Part model, mm, in its own coordinate system. A direction names the side the tool comes from. Round coordinates to 2 decimals unless told otherwise and drop trailing zeros. Loops run counter-clockwise (first coordinate to the right, second up) from the corner with the lowest first, then second, coordinate; pieces in that order, holes last. Notation, with made-up numbers: (78.25, 17) - (123.25, 17) arc R32 ccw to (123.25, 50) - close; hole circle Ø9 at (47, -8). An arc over 180 degrees is marked (long way). Write each question's results on one line, items separated by ' | '. Start each with the question number.
(1) Mould opens along X. For faces 4 (the face through (-90.49, -63, 1)), 5 (the face through (-105, -85.722, 1)), 6 (the face through (-107.615, -92, 1)) say: released by +X, released by -X, zero draft, split by the parting line, or undercut.
(2) Cut at A-A, the plane x = -114. List the corners of the cut face in (y, z), then the cut area to 3 significant figures.
(3) Cut at B-B, the plane y = -76. List the corners of the cut face in (x, z).
(4) Cut at D-D, the plane x = -88. List the corners of the cut face in (y, z).
(5) Cut at C-C, the plane z = 2. List the corners of the cut face in (x, y).
(6) Flat gauge pins, fed straight in: P1, Ø1.2, axis at x = -100.5, z = 1.5, coming from the +Y side; P2, Ø3, axis at x = -116.5, y = -84.5, coming from the -Z side; P3, Ø1.2, axis at y = -92.5, z = 1, coming from the +X side; P4, Ø1.2, axis at y = -91.5, z = 1.5, coming from the -X side. Where does each tip first touch, or does it go through?
(7) Tool access for faces 1 (the face through (-107.615, -63, 1)), 2 (the face through (-120.38, -70.12, 1.22)), 3 (the face through (-116, -90.722, 1)): list every direction of +Z, -Z, +X, -X, +Y, -Y with a clear straight run to the whole face (end or side of a thin tool).
(8) Drill centre lines: L1, parallel to Y at x = -98, z = 1.6; L2, parallel to X at y = -78, z = 1.8; L3, parallel to Y at x = -107.5, z = 2.25. Where is each one in solid material? Low to high.
from build123d import *

# Parameters (mm, degrees)
SALIENTE_EXTRUIR1_DEPTH = 2.4
CORTAR_EXTRUIR1_DEPTH   = 4


with BuildPart() as part:
    # Croquis1 → Saliente-Extruir1 (new body)
    with BuildSketch(Plane.XY):
        with BuildLine():
            Line((-102.615102368, -90.721952824), (-86.990102368, -90.721952824))
            ThreePointArc((-86.990102368, -90.721952824), (-84.868782024, -89.843273168), (-83.990102368, -87.721952824))
            Line((-83.990102368, -87.721952824), (-83.990102368, -67.221952824))
            ThreePointArc((-83.990102368, -67.221952824), (-84.868782024, -65.10063248), (-86.990102368, -64.221952824))
            Line((-86.990102368, -64.221952824), (-90.490102368, -64.221952824))
            Line((-90.490102368, -64.221952824), (-90.490102368, -61.221952824))
            Line((-90.490102368, -61.221952824), (-95.490102368, -61.221952824))
            Line((-95.490102368, -61.221952824), (-95.490102368, -64.221952824))
            Line((-95.490102368, -64.221952824), (-102.615102368, -64.221952824))
            Line((-102.615102368, -64.221952824), (-102.615102368, -61.221952824))
            Line((-102.615102368, -61.221952824), (-105.115102368, -61.221952824))
            Line((-105.115102368, -61.221952824), (-107.615102368, -61.221952824))
            Line((-107.615102368, -61.221952824), (-107.615102368, -64.221952824))
            Line((-107.615102368, -64.221952824), (-123.240102368, -64.221952824))
            ThreePointArc((-123.240102368, -64.221952824), (-125.361422711, -65.10063248), (-126.240102368, -67.221952824))
            Line((-126.240102368, -67.221952824), (-126.240102368, -87.721952824))
            ThreePointArc((-126.240102368, -87.721952824), (-125.361422711, -89.843273168), (-123.240102368, -90.721952824))
            Line((-123.240102368, -90.721952824), (-107.615102368, -90.721952824))
            Line((-107.615102368, -90.721952824), (-107.615102368, -93.721952824))
            Line((-107.615102368, -93.721952824), (-102.615102368, -93.721952824))
            Line((-102.615102368, -93.721952824), (-102.615102368, -90.721952824))
        make_face()
    extrude(amount=SALIENTE_EXTRUIR1_DEPTH)

    # Croquis2 → Cortar-Extruir1 (cut)
    with BuildSketch(Plane.XY.offset(2.4)):
        with BuildLine():
            Line((-115.427602368, -69.221952824), (-91.990102368, -69.221952824))
            ThreePointArc((-91.990102368, -69.221952824), (-89.868782024, -70.10063248), (-88.990102368, -72.221952824))
            Line((-88.990102368, -72.221952824), (-88.990102368, -82.721952824))
            ThreePointArc((-88.990102368, -82.721952824), (-89.868782024, -84.843273168), (-91.990102368, -85.721952824))
            Line((-91.990102368, -85.721952824), (-118.240102368, -85.721952824))
            ThreePointArc((-118.240102368, -85.721952824), (-120.361422711, -84.843273168), (-121.240102368, -82.721952824))
            Line((-121.240102368, -82.721952824), (-121.240102368, -72.221952824))
            ThreePointArc((-121.240102368, -72.221952824), (-120.361422711, -70.10063248), (-118.240102368, -69.221952824))
            Line((-118.240102368, -69.221952824), (-115.427602368, -69.221952824))
        make_face()
    extrude(amount=-CORTAR_EXTRUIR1_DEPTH, mode=Mode.SUBTRACT)


solid = part.part
A:
1) face 4: released by +X | face 5: undercut | face 6: released by -X
2) outline: (-90.72, 0) - (-85.72, 0) - (-85.72, 2.4) - (-90.72, 2.4) - close; (-69.22, 0) - (-64.22, 0) - (-64.22, 2.4) - (-69.22, 2.4) - close | area: 24.0 mm2
3) outline: (-126.24, 0) - (-121.24, 0) - (-121.24, 2.4) - (-126.24, 2.4) - close; (-88.99, 0) - (-83.99, 0) - (-83.99, 2.4) - (-88.99, 2.4) - close
4) outline: (-90.72, 0) - (-64.22, 0) - (-64.22, 2.4) - (-90.72, 2.4) - close
5) outline: (-126.24, -87.72) arc R3 ccw to (-123.24, -90.72) - (-107.62, -90.72) - (-107.62, -93.72) - (-102.62, -93.72) - (-102.62, -90.72) - (-86.99, -90.72) arc R3 ccw to (-83.99, -87.72) - (-83.99, -67.22) arc R3 ccw to (-86.99, -64.22) - (-90.49, -64.22) - (-90.49, -61.22) - (-95.49, -61.22) - (-95.49, -64.22) - (-102.62, -64.22) - (-102.62, -61.22) - (-107.62, -61.22) - (-107.62, -64.22) - (-123.24, -64.22) arc R3 ccw to (-126.24, -67.22) - close; hole (-121.24, -82.72) arc R3 ccw to (-118.24, -85.72) - (-91.99, -85.72) arc R3 ccw to (-88.99, -82.72) - (-88.99, -72.22) arc R3 ccw to (-91.99, -69.22) - (-118.24, -69.22) arc R3 ccw to (-121.24, -72.22) - close
6) P1: y = -64.22 | P2: z = 0 | P3: x = -102.62 | P4: x = -107.62
7) face 1: +Z, -Z, -X, +Y | face 2: +Z, -Z | face 3: +Z, -Z, -X, -Y
8) L1: -90.72 to -85.72, -69.22 to -64.22 | L2: -126.24 to -121.24, -88.99 to -83.99 | L3: -93.72 to -85.72, -69.22 to -61.22
